Read the model definition and answer for the solid it produces. Units are mm, in the model's axes. A direction names the side the tool comes from. Give positions to 0.01 mm unless a question says otherwise; leave off trailing zeros. Order: outer loops, then holes, each group sorted by start corner. A loop starts at its lowest first (then second) coordinate and runs counter-clockwise, first axis right, second up. Notation, with made-up numbers: (1.5, -37.75) - (60.5, -37.75) arc R7 cw to (60.5, -31.75) - close; hole circle Ø11 at (50, 28). An arc over 180 degrees is marked (long way). Write each question's results on one line, items separated by ' | '. Start each with the question number.
Q1. Flat-ended cylindrical pins translate along their axes: P1, Ø1.5, axis at y = 2.5, z = -1.5, coming from the -X side; P2, Ø0.6, axis at x = 4, y = 3, coming from the -Z side; P3, Ø0.6, axis at x = 4, y = 3.5, coming from the +Z side; P4, Ø1, axis at y = 3.5, z = -5.5, coming from the +X side. Find the tip coordinate at first contact, or state that the pin passes through.
Q2. Find section A-A on z = -4. Give the vertices of the cut face in (x, y), and give its area (4 significant figures).
Q3. Find section C-C on y = 2.8. Give the vertices of the cut face in (x, z).
Q4. Find the intervals of material crossed by line 1 along Y through (x, z) = (15, -8.5); line 2 along X through (y, z) = (3.15, -3); line 3 along Z through (x, y) = (6.5, 3.75), in increasing order. Write a range as from..to.
Q5. Find section B-B on x = 14.75. Give the vertices of the cut face in (y, z).
Q6. A tool of negligible diameter and unlimited length cuts with its end or side. For faces 1 (the face through (7.4, 3, -5)), 2 (the face through (2.6, 3, -5)), 3 (the face through (5, 3, -7.4)), from which of +Z, -Z, +X, -X, +Y, -Y can it reach the whole face along a straight path? Write none if from no direction.
from build123d import *

# Parameters (mm, degrees)
ESBO_O3_W                = 30
ESBO_O3_H                = 10
RESSALTO_EXTRUS_O3_DEPTH = 2
ESBO_O4_W                = 4.8
ESBO_O4_H                = 4.8
RESSALTO_EXTRUS_O4_DEPTH = 2.5
CHANFRO2_SIZE            = 0.5
FILETE5_R                = 2
FILETE6_R                = 2
FILETE7_R                = 2
FILETE8_R                = 2


with BuildPart() as part:
    # Esboço3 → Ressalto-extrusão3 (new body)
    with BuildSketch(Plane(origin=(0, 0, 0), x_dir=(1, 0, 0), z_dir=(0, 1, 0))):
        with Locations((15, 5)):
            Rectangle(ESBO_O3_W, ESBO_O3_H)
    extrude(amount=RESSALTO_EXTRUS_O3_DEPTH)

    # Esboço4 → Ressalto-extrusão4 (add)
    with BuildSketch(Plane(origin=(0, 2, 0), x_dir=(1, 0, 0), z_dir=(0, 1, 0))):
        with Locations((5, 5)):
            Rectangle(ESBO_O4_W, ESBO_O4_H)
    extrude(amount=RESSALTO_EXTRUS_O4_DEPTH)

    # Chanfro2
    chanfro2_edges = [part.edges().sort_by_distance(p)[0] for p in [
        (7.4, 2, -5),
        (5, 2, -7.4),
        (2.6, 2, -5),
        (5, 2, -2.6),
    ]]
    chamfer(chanfro2_edges, length=CHANFRO2_SIZE)

    # Filete5
    filete5_edges = [part.edges().sort_by_distance(p)[0] for p in [
        (0, 1, 0),
    ]]
    fillet(filete5_edges, radius=FILETE5_R)

    # Filete6
    filete6_edges = [part.edges().sort_by_distance(p)[0] for p in [
        (0, 1, -10),
    ]]
    fillet(filete6_edges, radius=FILETE6_R)

    # Filete7
    filete7_edges = [part.edges().sort_by_distance(p)[0] for p in [
        (30, 1, -10),
    ]]
    fillet(filete7_edges, radius=FILETE7_R)

    # Filete8
    filete8_edges = [part.edges().sort_by_distance(p)[0] for p in [
        (30, 1, 0),
    ]]
    fillet(filete8_edges, radius=FILETE8_R)


solid = part.part
Working result:
1) P1: x = 0 | P2: z = -7.4 | P3: z = -2.6 | P4: x = 7.4
2) outline: (0, 0) - (30, 0) - (30, 2) - (7.9, 2) - (7.4, 2.5) - (7.4, 4.5) - (2.6, 4.5) - (2.6, 2.5) - (2.1, 2) - (0, 2) - close | area: 72.25 mm²
3) outline: (2.6, -7.4) - (7.4, -7.4) - (7.4, -2.6) - (2.6, -2.6) - close
4) line 1: 0..2 | line 2: 2.6..7.4 | line 3: -7.4..-2.6
5) outline: (0, -10) - (2, -10) - (2, 0) - (0, 0) - close
6) face 1: +Z, -Z, +X, +Y | face 2: +Z, -Z, -X, +Y | face 3: -Z, +X, -X, +Y
